Can you work these out from the model? Positions are in its coordinate system, mm. Give positions to 0.01 mm unless a question says otherwise; leave off trailing zeros. Loops run counter-clockwise (first coordinate to the right, second up) from the corner with the lowest first, then second, coordinate; pieces in that order, holes last. Notation, with made-up numbers: (32, -37.5) - (62, -37.5) arc R27 cw to (62, -13.5) - close; hole circle Ø10 at (-21.5, -13). An arc over 180 degrees is marked (long way). Answer as a JSON object with one key per item and string values. Group by question number.
Item 1: Please list where these lines run through material, in increasing order: L1, parallel to X at y = 2.4, z = 21; L2, parallel to X at y = 1.2, z = 12; L3, parallel to Z at x = 44, y = 2.55 (3 decimals).
Item 2: Thinking about a two-plate mould opening in Z: for faces 1 (the cylindrical face through (195.039, 1.61, -20.315)), 2 (the cylindrical face through (170.743, 1.565, 22.549)), 3 (the flat face through (94, 0, 0)), which applies, pulls with the +Z half, pulls with the -Z half, needs draft (parallel to the pull), parting line crosses it, or undercut?
Item 3: Suppose I cut it at C-C on x = 50.8. Write out the boundary of the cut face in (y, z) (1 decimal).
Item 4: Will this pin go through, and if not, where does the flat tip stop? pin 1 (1.6 mm diameter, centred on x = 5, y = 1.5, fed in from -Z) (3 decimals).
Item 5: Suppose I cut it at B-B on z = 0. Count the separate pieces of the cut face and the enclosed holes in it, and give its area (3 significant figures).
Item 6: Suppose I cut it at A-A on x = 0. Write out the boundary of the cut face in (y, z) (3 decimals).
from build123d import *

# Parameters (mm, degrees)
SKETCH1_R           = 2.54
BOSS_EXTRUDE1_DEPTH = 3.175
SKETCH2_R           = 14.2875
CUT_EXTRUDE1_DEPTH  = 3.175
SKETCH3_R           = 2.54
CUT_EXTRUDE2_DEPTH  = 120.558881937
SKETCH5_R           = 2.4892
SKETCH5_R_2         = 2.54
BOSS_EXTRUDE2_DEPTH = 3.175
FILLET1_R           = 6.35


with BuildPart() as part:
    # Sketch1 → Boss-Extrude1 (new body)
    with BuildSketch(Plane(origin=(0, 0, 0), x_dir=(1, 0, 0), z_dir=(0, 1, 0))):
        Polygon((19.05, 15.875), (31.75, 34.925), (69.85, 34.925), (82.55, 15.875), (114.3, 15.875), (114.3, -15.875), (82.55, -15.875), (69.85, -34.925), (31.75, -34.925), (19.05, -15.875), (-12.7, -15.875), (-12.7, 15.875), align=None)
        with Locations(Location((0, 0, 0), (0, 0, 270))):
            Circle(SKETCH1_R, mode=Mode.SUBTRACT)
        with Locations(Location((101.6, 0, 0), (0, 0, 270))):
            Circle(SKETCH1_R, mode=Mode.SUBTRACT)
    extrude(amount=BOSS_EXTRUDE1_DEPTH)

    # Sketch2 → Cut-Extrude1 (cut)
    with BuildSketch(Plane(origin=(0, 3.175, 0), x_dir=(1, 0, 0), z_dir=(0, 1, 0))):
        with Locations(Location((50.8, 0, 0), (0, 0, 270))):
            Circle(SKETCH2_R)
    extrude(amount=-CUT_EXTRUDE1_DEPTH, mode=Mode.SUBTRACT)

    # Sketch3 → Cut-Extrude2 (cut, through all)
    with BuildSketch(Plane(origin=(0, 3.175, 0), x_dir=(1, 0, 0), z_dir=(0, 1, 0))):
        with Locations(Location((85.331391081, 0, 0), (0, 0, 270))):
            Circle(SKETCH3_R)
        with Locations(Location((16.268608919, 0, 0), (0, 0, 270))):
            Circle(SKETCH3_R)
    extrude(amount=-CUT_EXTRUDE2_DEPTH, mode=Mode.SUBTRACT)

    # Sketch5 → Boss-Extrude2 (add)
    with BuildSketch(Plane.XZ):
        Polygon((69.85, 34.925), (69.85, -34.925), (172.508333333, -34.925), (180.975, -22.225), (196.85, -22.225), (196.85, 22.225), (180.975, 22.225), (172.508333333, 34.925), align=None)
        with Locations(Location((130.175, -22.225, 0), (0, 0, 270))):
            Circle(SKETCH5_R, mode=Mode.SUBTRACT)
        with Locations(Location((168.275, -22.225, 0), (0, 0, 270))):
            Circle(SKETCH5_R, mode=Mode.SUBTRACT)
        with Locations(Location((85.331391081, 0, 0), (0, 0, 90))):
            Circle(SKETCH5_R_2, mode=Mode.SUBTRACT)
        with Locations(Location((101.6, 0, 0), (0, 0, 90))):
            Circle(SKETCH5_R_2, mode=Mode.SUBTRACT)
        with Locations(Location((130.175, 22.225, 0), (0, 0, 270))):
            Circle(SKETCH5_R, mode=Mode.SUBTRACT)
        with Locations(Location((190.5, 0, 0), (0, 0, 270))):
            Circle(SKETCH5_R_2, mode=Mode.SUBTRACT)
        with Locations(Location((168.275, 22.225, 0), (0, 0, 270))):
            Circle(SKETCH5_R, mode=Mode.SUBTRACT)
    extrude(amount=-BOSS_EXTRUDE2_DEPTH)

    # Fillet1
    fillet1_edges = [part.edges().sort_by_distance(p)[0] for p in [
        (19.05, 1.5875, -15.875),
        (31.75, 1.5875, -34.925),
        (31.75, 1.5875, 34.925),
        (19.05, 1.5875, 15.875),
        (-12.7, 1.5875, 15.875),
        (-12.7, 1.5875, -15.875),
        (172.508333333, 1.5875, 34.925),
        (172.508333333, 1.5875, -34.925),
        (180.975, 1.5875, -22.225),
        (196.85, 1.5875, -22.225),
        (196.85, 1.5875, 22.225),
        (180.975, 1.5875, 22.225),
    ]]
    fillet(fillet1_edges, radius=FILLET1_R)


solid = part.part
Worked out:
{
 "1": {"L1": "x = 22.47 to 128.01, 132.34 to 166.11, 170.44 to 194.25", "L2": "x = -12.2 to 43.05, 58.55 to 196.85", "L3": "z = -34.925 to -12.566, 12.566 to 34.925"},
 "2": {"face 1": "pulls with the -Z half", "face 2": "undercut", "face 3": "needs draft"},
 "3": {"outline": "(0, -34.9) - (3.2, -34.9) - (3.2, -14.3) - (0, -14.3) - close; (0, 14.3) - (3.2, 14.3) - (3.2, 34.9) - (0, 34.9) - close"},
 "4": {"pin 1": "stops at z = -15.875"},
 "5": {"separate pieces": "7", "enclosed holes": "0", "area": "494 mm2"},
 "6": {"outline": "(0, -15.875) - (3.175, -15.875) - (3.175, -2.54) - (0, -2.54) - close; (0, 2.54) - (3.175, 2.54) - (3.175, 15.875) - (0, 15.875) - close"}
}
